from build123d import *

# Parameters (mm, degrees)
SKETCH_1_W          = 30
SKETCH_1_H          = 10
EXTRUDE_1_DEPTH     = 4
SKETCH_2_W          = 2
SKETCH_2_H          = 15
CUT_EXTRUDE_1_DEPTH = 32.874754901
CUT_EXTRUDE_2_DEPTH = 32.874754901


with BuildPart() as part:
    # Эскиз1 → Бобышка-Вытянуть1 (new body)
    with BuildSketch(Plane(origin=(0, 0, 0), x_dir=(0, 0, -1), z_dir=(1, 0, 0))):
        with Locations((15, 5)):
            Rectangle(SKETCH_1_W, SKETCH_1_H)
    extrude(amount=EXTRUDE_1_DEPTH)

    # Эскиз2 → Вырез-Вытянуть1 (cut, through all)
    with BuildSketch(Plane(origin=(0, 10, 0), x_dir=(1, 0, 0), z_dir=(0, 1, 0))):
        with Locations((2, 13.5)):
            Rectangle(SKETCH_2_W, SKETCH_2_H)
    extrude(amount=-CUT_EXTRUDE_1_DEPTH, mode=Mode.SUBTRACT)

    # Эскиз3 → Вырез-Вытянуть2 (cut, through all)
    with BuildSketch(Plane(origin=(0, 10, 0), x_dir=(1, 0, 0), z_dir=(0, 1, 0))):
        Polygon((0, 23), (0, 30), (4, 30), align=None)
    extrude(amount=-CUT_EXTRUDE_2_DEPTH, mode=Mode.SUBTRACT)


solid = part.part
The listing builds one solid part. Answer for the finished solid, in the listing's coordinates (mm). A direction names the side the tool comes from. Round coordinates to 2 decimals unless told otherwise and drop trailing zeros. Write each loop counter-clockwise with the first axis right and the second up, starting at its lowest first coordinate (ties: lowest second). Pieces come first, ordered by that corner, then holes. Notation, with made-up numbers: M 69,31.25 L 94,31.25 A10 ccw 94,37.25 Z; hole C 32,76 d2. An arc over 180 degrees is marked long. Write each question's results on one line, items separated by ' | '. Start each with the question number.
Item 1: Find section A-A on y = 6. Write down the section's boundary in (x, z).
Item 2: Which of the six approach directions +Z, -Z, +X, -X, +Y, -Y give full straight-line access (tool end or side, diameter ignored) to faces 4 (the flat face through (0, 5, -11)), 5 (the flat face through (1, 5, -13))?
Item 3: Find section C-C on x = 1.4. Write down the section's boundary in (y, z).
Item 4: Find section D-D on x = 3.7. Write down the section's boundary in (y, z) (3 decimals), and give its area (3 significant figures).
Item 5: Straight lines are drawn through the part: probe 1 along X at (y, z) = (3.25, -9.75); probe 2 along Z at (x, y) = (1.55, 2.75); probe 3 along X at (y, z) = (6, -24.75). For each, find the intervals that lie inside material, in ascending order.
Item 6: Given pin 1 Ø2 at (x, y) = (2, 3.5) entering from -Z, flat-ended and moving along its own axis, determine where the tip first touches the part or whether it passes through.
Item 7: Find section B-B on z = -11. Write down the section's boundary in (x, y), and give its area (3 significant figures).
Item 8: The mould has two halves that part along Z. Classify faces 1 (the flat face through (3.3, 0, -14.8)), 2 (the flat face through (2, 5, 0)), 3 (the flat face through (2, 5, -21)): +Z half, -Z half, draft (parallel to the pull), parting line (faces both ways), or undercut.
Answer block:
1) outline: M 0,-23 L 4,-30 L 4,0 L 0,0 Z; hole M 1,-21 L 3,-21 L 3,-6 L 1,-6 Z
2) face 4: +Z, -Z, -X, +Y, -Y | face 5: +Y, -Y
3) outline: M 0,-25.45 L 10,-25.45 L 10,-21 L 0,-21 Z; M 0,-6 L 10,-6 L 10,0 L 0,0 Z
4) outline: M 0,-29.475 L 10,-29.475 L 10,0 L 0,0 Z | area: 295 mm²
5) probe 1: x = 0 to 1, 3 to 4 | probe 2: z = -25.71 to -21, -6 to 0 | probe 3: x = 1 to 4
6) pin 1: stops at z = -28.25
7) outline: M 0,0 L 1,0 L 1,10 L 0,10 Z; M 3,0 L 4,0 L 4,10 L 3,10 Z | area: 20.0 mm²
8) face 1: draft | face 2: +Z half | face 3: undercut
